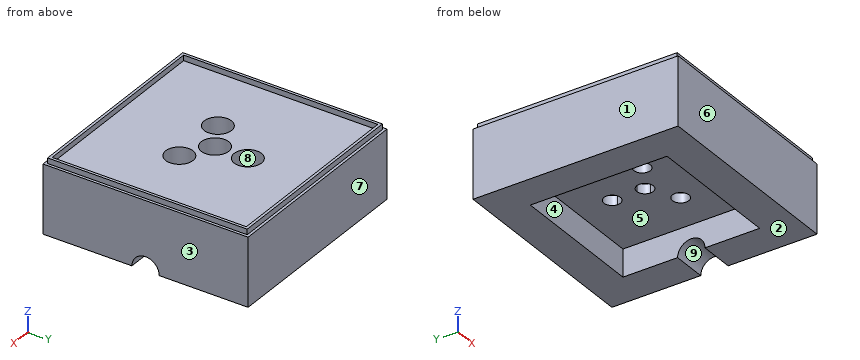
from build123d import *

# Parameters (mm, degrees)
F0_W      = 75
F0_H      = 75
F1_DEPTH  = 25
F2_W      = 73
F2_H      = 73
F2_W_2    = 71
F2_H_2    = 71
F3_DEPTH  = 2
F4_R      = 3
F5_DEPTH  = 20
F6_R      = 5
F7_DEPTH  = 11.5
F8_W      = 50
F8_H      = 50
F9_DEPTH  = 10
F10_R     = 5
F11_DEPTH = 15


with BuildPart() as f1:
    # F0 (on Top) → F1 (new body)
    with BuildSketch(Plane.XY):
        Rectangle(F0_W, F0_H)
    extrude(amount=F1_DEPTH)

    # F2 (on face) → F3 (join)
    with BuildSketch(Plane.XY.offset(25)):
        Rectangle(F2_W, F2_H)
        Rectangle(F2_W_2, F2_H_2, mode=Mode.SUBTRACT)
    extrude(amount=F3_DEPTH)

    # F4 (on face) → F5 (cut)
    with BuildSketch(Plane.XY.offset(25)):
        with BuildLine():
            ThreePointArc((0, 3), (-2.12132, -2.12132), (3, 0))
            ThreePointArc((3, 0), (2.12132, 2.12132), (0, 3))
        make_face()
        with BuildLine():
            ThreePointArc((3, 12), (-2.12132, 14.12132), (0, 9))
            ThreePointArc((0, 9), (2.12132, 9.87868), (3, 12))
        make_face()
        with Locations((-10.392305, -6)):
            Circle(F4_R)
        with Locations((10.392305, -6)):
            Circle(F4_R)
    extrude(amount=-F5_DEPTH, mode=Mode.SUBTRACT)

    # F6 (on face) → F7 (cut)
    with BuildSketch(Plane.XY.offset(25)):
        Circle(F6_R)
        with Locations((0, 12)):
            Circle(F6_R)
        with Locations((-10.392305, -6)):
            Circle(F6_R)
        with Locations((10.392305, -6)):
            Circle(F6_R)
    extrude(amount=-F7_DEPTH, mode=Mode.SUBTRACT)

    # F8 (on face) → F9 (cut)
    with BuildSketch(Plane(origin=(0, 0, 0), x_dir=(1, 0, 0), z_dir=(0, 0, -1))):
        Rectangle(F8_W, F8_H)
    extrude(amount=-F9_DEPTH, mode=Mode.SUBTRACT)

    # F10 (on face) → F11 (cut)
    with BuildSketch(Plane.YZ.offset(37.5)):
        Circle(F10_R)
    extrude(amount=-F11_DEPTH, mode=Mode.SUBTRACT)


solid = f1.part
CAD build for the part. Positions are in the model's coordinates, mm. Face numbers are marked on the shaded views. A direction names the side the tool comes from. Round coordinates to 2 decimals unless told otherwise and drop trailing zeros. Loops run counter-clockwise (first coordinate to the right, second up) from the corner with the lowest first, then second, coordinate; pieces in that order, holes last. Notation, with made-up numbers: M 8,76 L 28,76 A33 ccw 28,107 Z; hole C -13.75,34.5 d3. An arc over 180 degrees is marked long. One line per question, with ' | ' between items. Start each with the question number.
Item 1: Pin check, flat tips, straight feed: pin 1 Ø1 at (y, z) = (4.5, 26.5) entering from -X; pin 2 Ø3 at (x, y) = (25.5, 14) entering from +Z; pin 3 Ø9.5 at (x, y) = (10.39, -6) entering from -Z. Stop position of each tip, or through.
Item 2: Cut at C-C, the plane z = 6. Write the cut outline in (x, y).
Item 3: Wall check: line 1 (Y direction, x = 3, z = 3); line 2 (X direction, y = 0, z = 11.4); line 3 (X direction, y = -3, z = 24). Give the ranges that are in metal, low to high.
Item 4: Cut at D-D, the plane x = -18. Write the cut outline in (y, z).
Item 5: Which spindle directions (+Z, -Z, +X, -X, +Y, -Y) get a long thin tool onto all of the face, cutting with end or side? Do the marked faces 5, 6, 7, 8 and 9. Say none if no direction does.
Item 6: Cut at A-A, the plane z = 11. Write the cut outline in (x, y), plus the area to 3 significant figures.
Item 7: Cut at B-B, the plane y = -6. State how many separate pieces and enclosed holes the cut face has, plus the area to 3 significant figures.
Item 8: Two-plate mould, pull along X, no slides. Class the marked faces 1, 2, 3 and 4: pulls with the +X half, pulls with the -X half, needs draft (parallel to the pull), parting line crosses it, or undercut.
Responses:
1) pin 1: stops at x = -36.5 | pin 2: stops at z = 25 | pin 3: stops at z = 10
2) outline: M -37.5,-37.5 L 37.5,-37.5 L 37.5,37.5 L -37.5,37.5 Z; hole M -25,-25 L 25,-25 L 25,25 L -25,25 Z
3) line 1: y = -37.5 to -25, 25 to 37.5 | line 2: x = -37.5 to -3, 3 to 37.5 | line 3: x = -37.5 to -14.39, -6.39 to -4, 4 to 6.39, 14.39 to 37.5
4) outline: M -37.5,0 L -25,0 L -25,10 L 25,10 L 25,0 L 37.5,0 L 37.5,25 L 36.5,25 L 36.5,27 L 35.5,27 L 35.5,25 L -35.5,25 L -35.5,27 L -36.5,27 L -36.5,25 L -37.5,25 Z
5) face 5: -Z | face 6: +Z, -Z, +X, -X, -Y | face 7: +Z, -Z, +X, -X, +Y | face 8: +Z | face 9: -Z, +X
6) outline: M -37.5,-37.5 L 37.5,-37.5 L 37.5,37.5 L -37.5,37.5 Z; hole C -10.39,-6 d6; hole M 0,3 A3 ccw long 3,0 A3 ccw Z; hole M 0,9 A3 ccw 3,12 A3 ccw long Z; hole C 10.39,-6 d6 | area: 5,510 mm²
7) separate pieces: 3 | enclosed holes: 0 | area: 1,110 mm²
8) face 1: pulls with the -X half | face 2: needs draft | face 3: pulls with the +X half | face 4: undercut
